Autodesk Inventor part; units mm, degrees
ref_plane "YZ Plane" through (0, 0, 0) normal (1, 0, 0) x (0, 1, 0)
ref_plane "XZ Plane" through (0, 0, 0) normal (0, 1, 0) x (-1, 0, 0)
ref_plane "XY Plane" through (0, 0, 0) normal (0, 0, 1) x (1, 0, 0)
sketch "Sketch1" plane through (0, 0, 0) normal (0, 1, 0) x (-1, 0, 0)
  line L0 (12.5, 22.5) -> (-12.5, 22.5)
  line L1 (-12.5, 22.5) -> (-12.5, -22.5)
  line L2 (-12.5, -22.5) -> (12.5, -22.5)
  line L3 (12.5, -22.5) -> (12.5, 22.5)
  line L4 (12.5, 22.5) -> (-12.5, -22.5) construction
  line L5 (-12.5, 22.5) -> (12.5, -22.5) construction
  point P0 (0, 0)
  dimension "d0" = 25
  dimension "d1" = 45
extrude "Extrusion1" add sketch "Sketch1" along normal blind 32
sketch "Sketch2" plane through (0, 32, 0) normal (0, 1, 0) x (1, 0, 0)
  line L0 (12.5, -32) -> (-12.5, -32)
  line L1 (-12.5, -32) -> (-12.5, 32)
  line L2 (-12.5, 32) -> (12.5, 32)
  line L3 (12.5, 32) -> (12.5, -32)
  line L4 (12.5, -32) -> (-12.5, 32) construction
  line L5 (-12.5, -32) -> (12.5, 32) construction
  line L6 (0, -32) -> (0, -28)
  line L7 (0, 32) -> (0, 28)
  circle A0 centre (0, -28) radius 2
  circle A1 centre (0, 28) radius 2
  point P0 (0, 0)
  dimension "d4" = 64
  dimension "d5" = 4
  dimension "d6" = 4
  dimension "d7" = 4
  dimension "d8" = 4
extrude "Extrusion2" add sketch "Sketch2" along normal blind 5.2
sketch "Sketch3" plane through (0, 37.2, 0) normal (0, 1, 0) x (1, 0, 0)
  line L0 (12.5, 22.5) -> (-12.5, 22.5)
  line L1 (-12.5, -22.5) -> (12.5, -22.5)
  line L2 (12.5, -22.5) -> (12.5, 22.5)
  line L3 (12.5, 22.5) -> (-12.5, 22.5)
  line L4 (-12.5, 22.5) -> (-12.5, -22.5)
  line L5 (-12.5, -22.5) -> (12.5, 22.5) construction
  line L6 (12.5, -22.5) -> (-12.5, 22.5) construction
  point P0 (0, 0)
extrude "Extrusion3" add sketch "Sketch3" along normal blind 8
sketch "Sketch4" plane through (0, 45.2, 0) normal (0, 1, 0) x (1, 0, 0)
  line L0 (-12.5, 22.5) -> (-12.5, -22.5)
  line L1 (12.5, 22.5) -> (-12.5, 22.5)
  line L2 (12.5, -22.5) -> (12.5, 22.5)
  arc A0 (4.7196, -1.5748) -> (-4.7196, -1.5748) centre (0, 10) ccw
  line L3 (-12.5, 22.5) -> (12.5, 22.5)
  arc A1 (-4.7196, -1.5748) -> (4.7196, -1.5748) centre (0, -0.7) ccw
  point P0 (0, 0)
extrude "Extrusion4" add sketch "Sketch4" along normal blind 9 contours A0 A1
sketch "Sketch5" plane through (0, 54.2, 0) normal (0, 1, 0) x (1, 0, 0)
  arc A0 (4.7196, -1.5748) -> (-4.7196, -1.5748) centre (0, 10) ccw
  circle A1 centre (0, 10) radius 4.5
  point P0 (0, 0)
  dimension "d18" = 9
extrude "Extrusion5" add sketch "Sketch5" along normal blind 6
sketch "Sketch6" plane through (12.5, 0, -22.5) normal (0, 0, -1) x (-1, 0, 0)
  line L0 (8.5, 11) -> (16.5, 11)
  line L1 (16.5, 11) -> (16.5, 9)
  line L2 (16.5, 9) -> (8.5, 9)
  line L3 (8.5, 9) -> (8.5, 11)
  line L4 (8.5, 11) -> (16.5, 9) construction
  line L5 (16.5, 11) -> (8.5, 9) construction
  point P0 (12.5, 0)
  dimension "d22" = 8
  dimension "d23" = 2
extrude "Extrusion6" add sketch "Sketch6" along normal blind 10
scale "Scale1" factors (0.5, 0.5, 0.5) then translate (6.25, 8, -11.25) bodies 1
properties part number "Servo"
CAD build for the part. Positions are in the model's coordinates, mm. A direction names the side the tool comes from. Coordinates: 2 decimals unless noted, no trailing zeros. Write each loop counter-clockwise with the first axis right and the second up, starting at its lowest first coordinate (ties: lowest second). Pieces come first, ordered by that corner, then holes. Notation, with made-up numbers: (55, -14) - (84, -14) arc R16 ccw to (84, 15) - close; hole circle Ø2 at (73, 3). An arc over 180 degrees is marked (long way). Use a Markdown table: item, result. Add a question column.
Item 1: Band-saw the part on D-D, the plane x = 1. Give the cut face in (y, z), and give its area (3 significant figures).
Item 2: Band-saw the part on B-B, the plane z = -25.25. Give the cut face in (x, y).
Item 3: Flat gauge pins, fed straight in: pin 1 (7 mm diameter, centred on x = 3, z = -20, fed in from +Y); pin 2 (0.5 mm diameter, centred on y = 13, z = -25, fed in from -X); pin 3 (1.4 mm diameter, centred on x = 3.5, z = -24, fed in from -Y); pin 4 (1.4 mm diameter, centred on x = 4, z = -26, fed in from +Y). Where does each tip first touch, or does it go through?
Item 4: Drill centre lines: L1, parallel to Z at x = 6.25, y = 25.65; L2, parallel to X at y = 26.05, z = 2.75; L3, parallel to Z at x = 5.25, y = 11. Where is each one in solid material? Low to high. Write a range as from..to.
Item 5: Band-saw the part on C-C, the plane y = 27.5. Give the cut face in (x, z).
Item 6: Band-saw the part on A-A, the plane z = 2.75. Give the cut face in (x, y).
Item 7: Mould opens along Y. For faces 5 (the face through (5.513, 25.282, 3.426)), 6 (the face through (6, 24, 1)), 7 (the face through (6, 16, -22.5)) say: pulls with the +Y half, pulls with the -Y half, needs draft (parallel to the pull), parting line crosses it, or undercut.
Item 8: 3-axis set-ups, long thin cutter, end or side, ignore diameter. For faces 1 (the face through (6, 13.5, -25)), 2 (the face through (6.3, 32.8, -8.5)), 3 (the face through (4.25, 13, -25)), 4 (the face through (7.288, 36.579, -18.246)): which of +Z, -Z, +X, -X, +Y, -Y reach the whole face in a straight line?
Numbers:
| question | item | result |
|---|---|---|
| 1 | outline | (8, -22.5) - (24, -22.5) - (24, -27.25) - (26.6, -27.25) - (26.6, -22.5) - (30.6, -22.5) - (30.6, -19.64) - (35.1, -19.64) - (35.1, -12.86) - (30.6, -12.86) - (30.6, 0) - (26.6, 0) - (26.6, 4.75) - (24, 4.75) - (24, 0) - (8, 0) - close |
| 1 | area | 564 mm2 |
| 2 | outline | (0, 24) - (5.25, 24) - (5.25, 26.6) - (0, 26.6) - close; (4.25, 12.5) - (8.25, 12.5) - (8.25, 13.5) - (4.25, 13.5) - close; (7.25, 24) - (12.5, 24) - (12.5, 26.6) - (7.25, 26.6) - close |
| 3 | pin 1 | y = 38.1 |
| 3 | pin 2 | x = 4.25 |
| 3 | pin 3 | y = 24 |
| 3 | pin 4 | y = 26.6 |
| 4 | L1 | -27.25..-26.25, -24.25..1.75, 3.75..4.75 |
| 4 | L2 | 0..5.25, 7.25..12.5 |
| 4 | L3 | -22.5..0 |
| 5 | outline | (0, -22.5) - (12.5, -22.5) - (12.5, 0) - (0, 0) - close |
| 6 | outline | (0, 24) - (5.25, 24) - (5.25, 26.6) - (0, 26.6) - close; (7.25, 24) - (12.5, 24) - (12.5, 26.6) - (7.25, 26.6) - close |
| 7 | face 5 | needs draft |
| 7 | face 6 | pulls with the -Y half |
| 7 | face 7 | undercut |
| 8 | face 1 | -Z, +X, -X |
| 8 | face 2 | +Z, +Y |
| 8 | face 3 | -Z, -X, -Y |
| 8 | face 4 | +Y |
